```python
from build123d import *

# Parameters (mm, degrees)
F0_W      = 40
F0_H      = 40
F1_DEPTH  = 120
F2_W      = 40
F2_H      = 40
F2_R      = 17.5
F3_DEPTH  = 50
F4_R      = 5.5
F5_DEPTH  = 100
F6_W      = 20
F6_H      = 40
F7_DEPTH  = 50
F8_R      = 10
F9_DEPTH  = 15
F10_R     = 8
F11_DEPTH = 60


with BuildPart() as f1:
    # F0 (on Right) → F1 (new body)
    with BuildSketch(Plane.YZ):
        Rectangle(F0_W, F0_H)
    extrude(amount=-F1_DEPTH)

    # F2 (on face) → F3 (cut)
    with BuildSketch(Plane.YZ):
        Rectangle(F2_W, F2_H)
        Circle(F2_R, mode=Mode.SUBTRACT)
    extrude(amount=-F3_DEPTH, mode=Mode.SUBTRACT)

    # F4 (on face) → F5 (cut)
    with BuildSketch(Plane.YZ):
        Circle(F4_R)
    extrude(amount=-F5_DEPTH, mode=Mode.SUBTRACT)

    # F6 (on face) → F7 (cut)
    with BuildSketch(Plane(origin=(-120, 0, 0), x_dir=(0, -1, 0), z_dir=(-1, 0, 0))):
        Rectangle(F6_W, F6_H)
    extrude(amount=-F7_DEPTH, mode=Mode.SUBTRACT)

    # F8 (on face) → F9 (cut)
    with BuildSketch(Plane(origin=(-70, 0, 0), x_dir=(0, -1, 0), z_dir=(-1, 0, 0))):
        Circle(F8_R)
    extrude(amount=-F9_DEPTH, mode=Mode.SUBTRACT)

    # F10 (on face) → F11 (cut, symmetric)
    with BuildSketch(Plane.XZ.offset(20)):
        with Locations((-100, 0)):
            Circle(F10_R)
    extrude(amount=F11_DEPTH, both=True, mode=Mode.SUBTRACT)


solid = f1.part
```
Could you check a few things on this model? Use its own coordinates, in mm. A direction names the side the tool comes from. Round coordinates to 2 decimals unless told otherwise and drop trailing zeros. Loops run counter-clockwise (first coordinate to the right, second up) from the corner with the lowest first, then second, coordinate; pieces in that order, holes last. Notation, with made-up numbers: (78, 23.5) -> (97, 23.5) arc R33 cw to (97, 56.5) -> close; hole circle Ø10 at (26.25, -24). An arc over 180 degrees is marked (long way). One line per question, with ' | ' between items.
(1) If we section it at C-C on y = 0: List the corners of the cut face in (x, z) for me, and give its area (4 significant figures).
Model answer:
outline: (-70, -20) -> (-50, -20) -> (-50, -17.5) -> (0, -17.5) -> (0, -5.5) -> (-55, -5.5) -> (-55, -10) -> (-70, -10) -> close; (-70, 10) -> (-55, 10) -> (-55, 5.5) -> (0, 5.5) -> (0, 17.5) -> (-50, 17.5) -> (-50, 20) -> (-70, 20) -> close | area: 1,645 mm^2
(2) For faces 5 (the face through (-50, -18, 0)), 6 (the face through (-62.6, 2.17, -9.76)), 7 (the face through (-90, -10, 0)), which set-ups out of +Z, -Z, +X, -X, +Y, -Y let a thin tool reach every point of the face, with its end or its side?
Model answer:
face 5: +X | face 6: -X | face 7: +Z, -Z, -X
(3) For pin 1 Ø21 at (x, z) = (-100, 0) entering from +Y; pin 2 Ø6.5 at (y, z) = (0, 0) entering from +X; pin 3 Ø1 at (y, z) = (7.5, 5) entering from -X; pin 4 Ø10 at (y, z) = (-2, 14.5) entering from -X, each with a flat end and sliding along its axis, tell me the tip position at first contact or that it passes through.
Model answer:
pin 1: stops at y = 20 | pin 2: passes through | pin 3: stops at x = -55 | pin 4: stops at x = -70
(4) If we section it at B-B on x = -84.5: List the corners of the cut face in (y, z) for me, and give its area (3 significant figures).
Model answer:
outline: (-20, -20) -> (-10, -20) -> (-10, 20) -> (-20, 20) -> close; (10, -20) -> (20, -20) -> (20, 20) -> (10, 20) -> close | area: 800 mm^2
(5) If we section it at D-D on y = 13: List the corners of the cut face in (x, z) for me, and give its area (3 significant figures).
Model answer:
outline: (-120, -20) -> (-50, -20) -> (-50, -11.72) -> (0, -11.72) -> (0, 11.72) -> (-50, 11.72) -> (-50, 20) -> (-120, 20) -> close; hole circle Ø16 at (-100, 0) | area: 3,770 mm^2
(6) Thinking about a two-plate mould opening in Z: for faces 1 (the face through (0, -4, -4)), 2 (the face through (-24.65, -13.887, -10.648)), 3 (the face through (-27.12, -1.19, -5.37)), 4 (the face through (-108, 15, 0)), which applies, released by +Z, released by -Z, zero draft, split by the parting line, or undercut?
Model answer:
face 1: zero draft | face 2: split by the parting line | face 3: undercut | face 4: undercut
(7) If I drill on probe 1 along Z at (x, y) = (-100, -17); probe 2 along Z at (x, y) = (-18.5, -0.5); probe 3 along Y at (x, z) = (-90, 8), over which ranges is the centre line in solid material (lowest first)?
Model answer:
probe 1: z = -20 to -8, 8 to 20 | probe 2: z = -17.49 to -5.48, 5.48 to 17.49 | probe 3: y = -20 to -10, 10 to 20
(8) If we section it at A-A on x = -100: List the corners of the cut face in (y, z) for me, and give its area (3 significant figures).
Model answer:
outline: (-20, -20) -> (-10, -20) -> (-10, -8) -> (-20, -8) -> close; (-20, 8) -> (-10, 8) -> (-10, 20) -> (-20, 20) -> close; (10, -20) -> (20, -20) -> (20, -8) -> (10, -8) -> close; (10, 8) -> (20, 8) -> (20, 20) -> (10, 20) -> close | area: 480 mm^2
